from build123d import *

# Parameters (mm, degrees)
SKETCH_R           = 50
SKETCH_R_2         = 7.5
PAD_DEPTH          = 20
SKETCH001_R        = 48.5
SKETCH001_R_2      = 8.25
POCKET_DEPTH       = 18.5
POCKET001_DEPTH    = 5
POLARPATTERN_COUNT = 4


with BuildPart() as part:
    # Sketch → Pad (new body)
    with BuildSketch(Plane.XY):
        Circle(SKETCH_R)
        Circle(SKETCH_R_2, mode=Mode.SUBTRACT)
    extrude(amount=PAD_DEPTH)

    # Sketch001 (on Face4 of Pad) → Pocket (cut)
    with BuildSketch(Plane.XY.offset(20)):
        Circle(SKETCH001_R)
        Circle(SKETCH001_R_2, mode=Mode.SUBTRACT)
    extrude(amount=-POCKET_DEPTH, mode=Mode.SUBTRACT)

    # Sketch002 (on Face2 of Pocket) → Pocket001 (cut)
    with BuildSketch(Plane(origin=(0, 0, 0), x_dir=(1, 0, 0), z_dir=(0, 0, -1))):
        with BuildLine():
            ThreePointArc((0, 46), (-7.791201, 45.335386), (-15.357265, 43.360747))
            Line((-15.357265, 43.360747), (-3.713796, 9.284811))
            ThreePointArc((0, 10), (-1.891017, 9.819575), (-3.713796, 9.284811))
            Line((0, 46), (0, 10))
        make_face()
    pocket001 = extrude(amount=-POCKET001_DEPTH, mode=Mode.SUBTRACT)

    # PolarPattern: Pocket001 ×4 about axis
    polarpattern_axis = Axis((0, 0, 0), (0, 0, -1))
    for i in range(1, POLARPATTERN_COUNT):
        add(pocket001.rotate(polarpattern_axis, i * 360 / POLARPATTERN_COUNT), mode=Mode.SUBTRACT)


solid = part.part
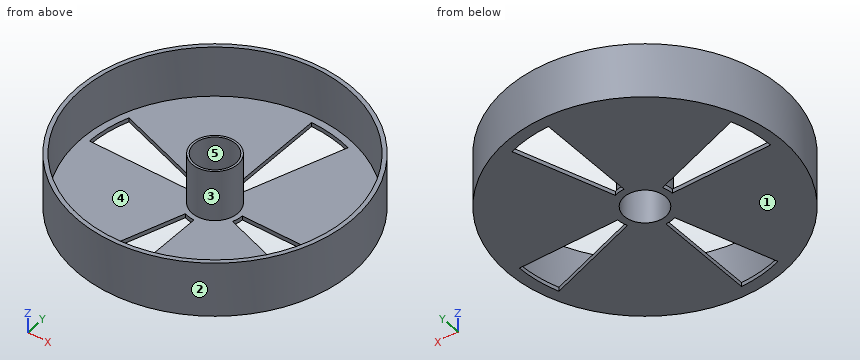
Geometry: final body of the model. Coordinates: model frame, mm. Face numbers are marked on the shaded views. A direction names the side the tool comes from. Give positions to 0.01 mm unless a question says otherwise; leave off trailing zeros. Loops run counter-clockwise (first coordinate to the right, second up) from the corner with the lowest first, then second, coordinate; pieces in that order, holes last. Notation, with made-up numbers: (20.5, 69.25) -> (40.5, 69.25) arc R30 cw to (40.5, 107.25) -> close; hole circle Ø9 at (-31.75, 33.5). An arc over 180 degrees is marked (long way). Put each result on its own line as item: value.
1. Cut plane B-B (x = 17). Return the cut outline in (y, z), plus the area to 3 significant figures.
Taken from the geometry:
outline: (-47.02, 0) -> (-6.35, 0) -> (-6.35, 1.5) -> (-45.42, 1.5) -> (-45.42, 20) -> (-47.02, 20) -> close; (0, 0) -> (47.02, 0) -> (47.02, 20) -> (45.42, 20) -> (45.42, 1.5) -> (0, 1.5) -> close
area: 191 mm2
2. Pull-direction query (X, two-part tool) for the marked faces 1, 2 and 3; classes: released by +X, released by -X, zero draft, split by the parting line, or undercut.
Taken from the geometry:
face 1: zero draft
face 2: split by the parting line
face 3: undercut
3. Set-up query: the marked faces 4 and 5. Return all of +Z, -Z, +X, -X, +Y, -Y with unobstructed straight access to the full face (end or side cutting, diameter ignored); none if empty.
Taken from the geometry:
face 4: +Z
face 5: +Z, -Z
4. Cut plane C-C (y = -19). Return the cut outline in (x, z), plus the area to 3 significant figures.
Taken from the geometry:
outline: (-46.25, 0) -> (-7.03, 0) -> (-7.03, 1.5) -> (-44.62, 1.5) -> (-44.62, 20) -> (-46.25, 20) -> close; (0, 0) -> (46.25, 0) -> (46.25, 20) -> (44.62, 20) -> (44.62, 1.5) -> (0, 1.5) -> close
area: 188 mm2
5. Pin query (flat end, axial travel): P1, Ø12, axis at x = 0, y = 0, coming from the -Z side; P2, Ø1.6, axis at x = -27.5, z = 1, coming from the +Y side; P3, Ø1, axis at x = -15.5, z = 10.5, coming from the +Y side; P4, Ø10, axis at x = 27, z = 18, coming from the -Y side. Return the tip coordinate at first contact, or that it passes through.
Taken from the geometry:
P1: passes through
P2: stops at y = 42.27
P3: stops at y = 47.7
P4: stops at y = -44.9
6. Ray query, line 1 along Y through (x, z) = (0, 6.25); line 2 along Y through (x, z) = (-1.5, 14.75); line 3 along Z through (x, y) = (42.5, 9). Return the intervals inside material, ascending. Write a range as [from, to].
Taken from the geometry:
line 1: y = [-50, -48.5], [-8.25, -7.5], [7.5, 8.25], [48.5, 50]
line 2: y = [-49.98, -48.48], [-8.11, -7.35], [7.35, 8.11], [48.48, 49.98]
line 3: z = [0, 1.5]
7. Cut plane A-A (z = 5.75). Return the cut outline in (x, y).
Taken from the geometry:
outline: circle Ø100 at (0, 0); circle Ø16.5 at (0, 0); hole circle Ø97 at (0, 0); hole circle Ø15 at (0, 0)
